Part print with two shaded views. Sizes in mm from the minimum x, y, z corner. Coordinates: 2 decimals unless noted, no trailing zeros. Order: outer loops, then holes, each group sorted by start corner. A loop starts at its lowest first (then second) coordinate and runs counter-clockwise, first axis right, second up. Notation, with made-up numbers: (-40, 19.25) - (12, 19.25) arc R27 ccw to (12, 47.25) - close; hole circle Ø1 at (-2.5, 19). An arc over 180 degrees is marked (long way). One line per item, written item: value.
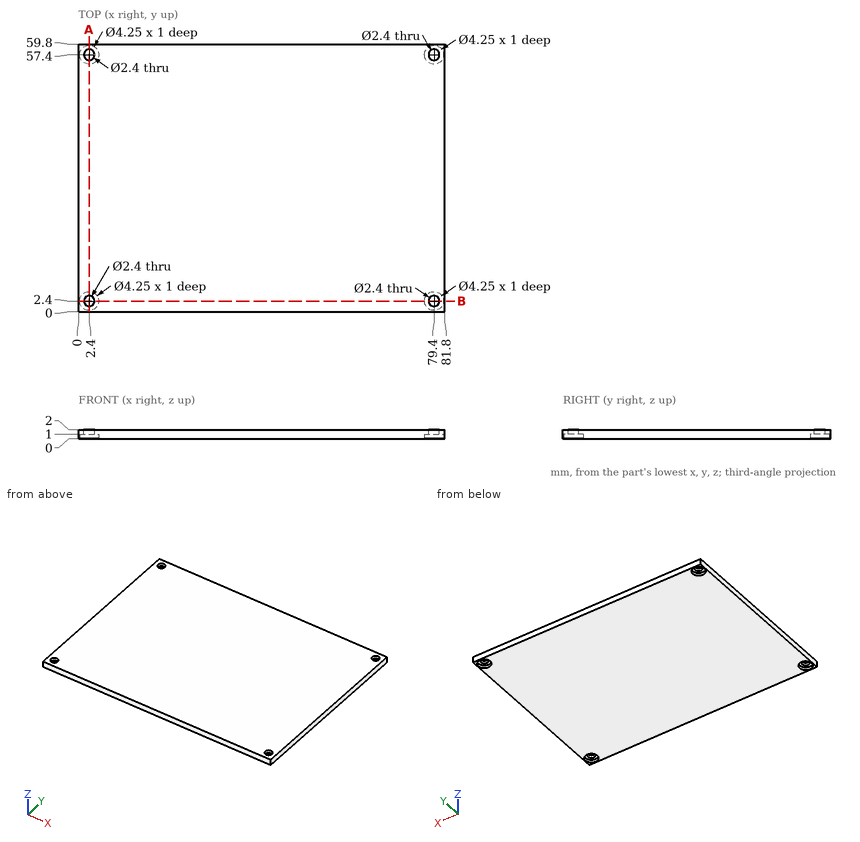
1. Band-saw the part on B-B, the plane y = 2.4. Give the cut face in (x, z) (3 decimals), and give its area (3 significant figures).
Values found:
outline: (0, 0) - (0.275, 0) - (0.275, 1) - (1.2, 1) - (1.2, 2) - (0, 2) - close; (3.6, 1) - (4.525, 1) - (4.525, 0) - (77.275, 0) - (77.275, 1) - (78.2, 1) - (78.2, 2) - (3.6, 2) - close; (80.6, 1) - (81.525, 1) - (81.525, 0) - (81.8, 0) - (81.8, 2) - (80.6, 2) - close
area: 150 mm2
2. Band-saw the part on A-A, the plane x = 2.4. Give the cut face in (y, z) (3 decimals), and give its area (3 significant figures).
Values found:
outline: (0, 0) - (0.275, 0) - (0.275, 1) - (1.2, 1) - (1.2, 2) - (0, 2) - close; (3.6, 1) - (4.525, 1) - (4.525, 0) - (55.275, 0) - (55.275, 1) - (56.2, 1) - (56.2, 2) - (3.6, 2) - close; (58.6, 1) - (59.525, 1) - (59.525, 0) - (59.8, 0) - (59.8, 2) - (58.6, 2) - close
area: 106 mm2
3. Probe line 1 along Y through (x, z) = (2.4, 1.65); line 2 along Y through (x, z) = (2.4, 0.35) (3 decimals). List the from-to ranges inside material, lowest first.
Values found:
line 1: y = 0 to 1.2, 3.6 to 56.2, 58.6 to 59.8
line 2: y = 0 to 0.275, 4.525 to 55.275, 59.525 to 59.8
4. Flat gauge pin, fed straight in: P1, Ø2, axis at x = 79, y = 1.5, coming from the -Z side. Where does the tip first touch, or does it go through?
Values found:
P1: stops at z = 1
